Could you check a few things on this model? Use its own coordinates, in mm. Face numbers are marked on the shaded views. Give positions to 0.01 mm unless a question says otherwise; leave off trailing zeros. Write each loop counter-clockwise with the first axis right and the second up, starting at its lowest first coordinate (ties: lowest second). Pieces come first, ordered by that corner, then holes. Notation, with made-up numbers: (-36, 43) - (-26, 43) arc R16 cw to (-26, 56) - close; hole circle Ø10 at (81.5, 66.25). An arc over 180 degrees is marked (long way). Write item = value, one per line.
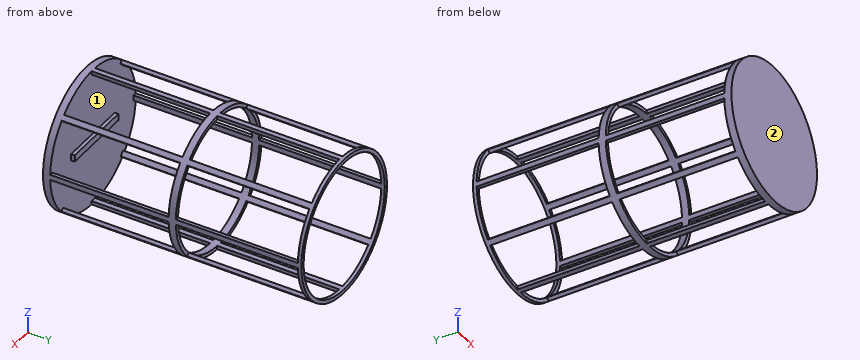
from build123d import *

# Parameters (mm, degrees)
SKETCH1_R               = 49.53
SKETCH1_R_2             = 46.99
BOSS_EXTRUDE1_DEPTH     = 182.88
CUT_EXTRUDE1_DEPTH      = 177.8
SKETCH3_R               = 49.53
SKETCH3_R_2             = 46.99
BOSS_EXTRUDE2_DEPTH     = 2.54
SKETCH4_R               = 49.53
SKETCH4_R_2             = 46.99
BOSS_EXTRUDE3_DEPTH     = 2.54
BOSS_EXTRUDE4_START     = -5.08
SKETCH5_R               = 49.53
BOSS_EXTRUDE4_DEPTH     = 5.08
SKETCH6_W               = 50.419
SKETCH6_H               = 4.699
BOSS_EXTRUDE5_DEPTH     = 2.54
SKETCH7_R               = 0.8255
BOSS_EXTRUDE6_DEPTH     = 2.54
CIRPATTERN2_COUNT       = 8
CUT_EXTRUDE2_DEPTH      = 199.209531052
CUT_EXTRUDE2_DEPTH_BACK = 199.209531052
SKETCH8_W               = 111.115562831
SKETCH8_H               = 193.581618433


with BuildPart() as part:
    # Sketch1 → Boss-Extrude1 (new, symmetric)
    with BuildSketch(Plane(origin=(0, 0, 0), x_dir=(1, 0, 0), z_dir=(0, 1, 0))):
        with Locations(Location((0, 0, 0), (0, 0, 270))):
            Circle(SKETCH1_R)
        with Locations(Location((0, 0, 0), (0, 0, 270))):
            Circle(SKETCH1_R_2, mode=Mode.SUBTRACT)
    extrude(amount=BOSS_EXTRUDE1_DEPTH, both=True)

    # Sketch2 → Cut-Extrude1 (cut, symmetric)
    with BuildSketch(Plane(origin=(0, 0, 0), x_dir=(1, 0, 0), z_dir=(0, 1, 0))):
        with BuildLine():
            Line((34.339077963, -32.07628134), (36.13611782, -33.873321197))
            ThreePointArc((36.13611782, -33.873321197), (45.710930003, -19.071753413), (49.49527883, -1.854258207))
            Line((49.49527883, -1.854258207), (46.953400585, -1.854258207))
            ThreePointArc((46.953400585, -1.854258207), (43.364264524, -18.099742051), (34.339077963, -32.07628134))
        make_face()
        with BuildLine():
            ThreePointArc((1.584890151, -49.504636381), (18.664975227, -45.878530924), (33.425440685, -36.550797734))
            Line((33.425440685, -36.550797734), (31.627502039, -34.752859088))
            ThreePointArc((31.627502039, -34.752859088), (17.692915235, -43.531837205), (1.584890151, -46.963264614))
            Line((1.584890151, -46.963264614), (1.584890151, -49.504636381))
        make_face()
        with BuildLine():
            ThreePointArc((-33.543952964, -36.442065248), (-19.03558139, -45.726005086), (-2.225109849, -49.479993797))
            Line((-2.225109849, -49.479993797), (-2.225109849, -46.937287801))
            ThreePointArc((-2.225109849, -46.937287801), (-18.063572268, -43.379343666), (-31.746279167, -34.644391451))
            Line((-31.746279167, -34.644391451), (-33.543952964, -36.442065248))
        make_face()
        with BuildLine():
            Line((46.949282998, 1.955741793), (49.491372723, 1.955741793))
            ThreePointArc((49.491372723, 1.955741793), (45.777644234, 18.911059948), (36.442065248, 33.543952964))
            Line((36.442065248, 33.543952964), (34.644391451, 31.746279167))
            ThreePointArc((34.644391451, 31.746279167), (43.430990742, 17.93903964), (46.949282998, 1.955741793))
        make_face()
        with BuildLine():
            ThreePointArc((-49.49527883, -1.854258207), (-45.741824116, -18.997537381), (-36.245883162, -33.755841773))
            Line((-36.245883162, -33.755841773), (-34.448634556, -31.958593167))
            ThreePointArc((-34.448634556, -31.958593167), (-43.39516767, -18.025524205), (-46.953400585, -1.854258207))
            Line((-46.953400585, -1.854258207), (-49.49527883, -1.854258207))
        make_face()
        with BuildLine():
            Line((31.958593167, 34.448634556), (33.755841773, 36.245883162))
            ThreePointArc((33.755841773, 36.245883162), (18.873008967, 45.79334485), (1.584890151, 49.504636381))
            Line((1.584890151, 49.504636381), (1.584890151, 46.963264614))
            ThreePointArc((1.584890151, 46.963264614), (17.900986276, 43.446689061), (31.958593167, 34.448634556))
        make_face()
        with BuildLine():
            ThreePointArc((-36.550797734, 33.425440685), (-45.80828813, 18.836709868), (-49.491372723, 1.955741793))
            Line((-49.491372723, 1.955741793), (-46.949282998, 1.955741793))
            ThreePointArc((-46.949282998, 1.955741793), (-43.461630715, 17.864678995), (-34.752859088, 31.627502039))
            Line((-34.752859088, 31.627502039), (-36.550797734, 33.425440685))
        make_face()
        with BuildLine():
            Line((-2.225109849, 46.937287801), (-2.225109849, 49.479993797))
            ThreePointArc((-2.225109849, 49.479993797), (-19.242893169, 45.63914945), (-33.873321197, 36.13611782))
            Line((-33.873321197, 36.13611782), (-32.07628134, 34.339077963))
            ThreePointArc((-32.07628134, 34.339077963), (-18.270880717, 43.292436035), (-2.225109849, 46.937287801))
        make_face()
    extrude(amount=CUT_EXTRUDE1_DEPTH, both=True, mode=Mode.SUBTRACT)

    # Sketch3 → Boss-Extrude2 (add, symmetric)
    with BuildSketch(Plane(origin=(0, 91.44, 0), x_dir=(1, 0, 0), z_dir=(0, 1, 0))):
        with Locations(Location((0, 0, 0), (0, 0, 270))):
            Circle(SKETCH3_R)
        with Locations(Location((0, 0, 0), (0, 0, 270))):
            Circle(SKETCH3_R_2, mode=Mode.SUBTRACT)
    boss_extrude2 = extrude(amount=BOSS_EXTRUDE2_DEPTH, both=True)

    # Mirror1: Boss-Extrude2 across plane
    add(boss_extrude2.mirror(Plane.ZX))

    # Sketch4 → Boss-Extrude3 (add, symmetric)
    with BuildSketch(Plane(origin=(0, 0, 0), x_dir=(1, 0, 0), z_dir=(0, 1, 0))):
        with Locations(Location((0, 0, 0), (0, 0, 270))):
            Circle(SKETCH4_R)
        with Locations(Location((0, 0, 0), (0, 0, 270))):
            Circle(SKETCH4_R_2, mode=Mode.SUBTRACT)
    extrude(amount=BOSS_EXTRUDE3_DEPTH, both=True)

    # Sketch5 → Boss-Extrude4 (add)
    with BuildSketch(Plane.XZ.offset(182.88).offset(BOSS_EXTRUDE4_START)):
        with Locations(Location((0, 0, 0), (0, 0, 90))):
            Circle(SKETCH5_R)
    extrude(amount=BOSS_EXTRUDE4_DEPTH)

    # Sketch6 → Boss-Extrude5 (add)
    with BuildSketch(Plane(origin=(0, -177.8, 0), x_dir=(1, 0, 0), z_dir=(0, 1, 0))):
        Rectangle(SKETCH6_W, SKETCH6_H)
    extrude(amount=BOSS_EXTRUDE5_DEPTH)

    # Sketch7 → Boss-Extrude6 (add)
    with BuildSketch(Plane(origin=(0, 182.88, 0), x_dir=(1, 0, 0), z_dir=(0, 1, 0))):
        with Locations(Location((48.26, 0, 0), (0, 0, 270))):
            Circle(SKETCH7_R)
    boss_extrude6 = extrude(amount=BOSS_EXTRUDE6_DEPTH)

    # CirPattern2: Boss-Extrude6 ×8 about axis
    cirpattern2_axis = Axis((0, 0, 0), (0, 1, 0))
    for i in range(1, CIRPATTERN2_COUNT):
        add(boss_extrude6.rotate(cirpattern2_axis, i * 360 / CIRPATTERN2_COUNT))

    # Sketch8 → Cut-Extrude2 (cut, two sides: drawn at the far end of the back side and taken through both)
    with BuildSketch(Plane.XY.offset(-CUT_EXTRUDE2_DEPTH_BACK)):
        with Locations((1.84635432, 96.790809217)):
            Rectangle(SKETCH8_W, SKETCH8_H)
    extrude(amount=CUT_EXTRUDE2_DEPTH + CUT_EXTRUDE2_DEPTH_BACK, mode=Mode.SUBTRACT)


solid = part.part
1. If we section it at B-B, the plane z = -24: Please give me the cut outline in (x, y).
Filled sheet:
outline = (-43.33, -182.88) - (43.33, -182.88) - (43.33, -177.8) - (-43.33, -177.8) - close; (-43.33, -93.98) - (-40.4, -93.98) - (-40.4, -88.9) - (-43.33, -88.9) - close; (-43.33, -2.54) - (-40.4, -2.54) - (-40.4, 0) - (-43.33, 0) - close; (40.4, -93.98) - (43.33, -93.98) - (43.33, -88.9) - (40.4, -88.9) - close; (40.4, -2.54) - (43.33, -2.54) - (43.33, 0) - (40.4, 0) - close
2. Thinking about a two-plate mould opening in Z: for the marked faces 1 and 2, which applies, pulls with the +Z half, pulls with the -Z half, needs draft (parallel to the pull), parting line crosses it, or undercut?
Filled sheet:
face_1 = undercut
face_2 = needs draft
3. If we section it at A-A, the plane y = -34: Count the separate pieces of the cut face and the enclosed holes in it, and give its area (3 significant figures).
Filled sheet:
separate_pieces = 8
enclosed_holes = 0
area = 77.4 mm2
4. I need wall thicknesses on line 1 (Y direction, x = 25.5, z = 40); line 2 (X direction, y = -71, z = -0.5); line 3 (Y direction, x = 14.5, z = 42). Which ranges of each line are inside material? Lowest first, please.
Filled sheet:
line_1 = -182.88 to -177.8, -93.98 to -88.9, -2.54 to 0
line_2 = -49.53 to -46.99, 46.99 to 49.53
line_3 = -182.88 to -177.8
5. If we section it at C-C, the plane z = 0: Please give me the cut outline in (x, y), and give its area (3 significant figures).
Filled sheet:
outline = (-49.53, -182.88) - (49.53, -182.88) - (49.53, 0) - (46.99, 0) - (46.99, -177.8) - (25.21, -177.8) - (25.21, -175.26) - (-25.21, -175.26) - (-25.21, -177.8) - (-46.99, -177.8) - (-46.99, 0) - (-49.53, 0) - close
area = 1,530 mm2
6. For pin 1 (3 mm diameter, centred on x = -48, y = -149, fed in from -Z); pin 2 (1.5 mm diameter, centred on x = -30.5, y = -62, fed in from -Z); pin 3 (1.3 mm diameter, centred on y = -132.5, z = 48.5, fed in from -X); pin 4 (8 mm diameter, centred on x = 38.5, y = -30, fed in from +Z), each with a flat end and sliding along its axis, tell me the tip position at first contact or that it passes through.
Filled sheet:
pin_1 = -1.96
pin_2 = through
pin_3 = -2.23
pin_4 = 35.54
7. If we section it at D-D, the plane z = -39: Please give me the cut outline in (x, y).
Filled sheet:
outline = (-30.53, -182.88) - (30.53, -182.88) - (30.53, -177.8) - (-30.53, -177.8) - close; (-30.53, -93.98) - (-26.21, -93.98) - (-26.21, -88.9) - (-30.53, -88.9) - close; (-30.53, -2.54) - (-26.21, -2.54) - (-26.21, 0) - (-30.53, 0) - close; (26.21, -93.98) - (30.53, -93.98) - (30.53, -88.9) - (26.21, -88.9) - close; (26.21, -2.54) - (30.53, -2.54) - (30.53, 0) - (26.21, 0) - close
